Build history of the part. All positions in model axes, mm. Face numbers are marked on the shaded views. Give positions to 0.01 mm unless a question says otherwise; leave off trailing zeros. Order: outer loops, then holes, each group sorted by start corner. A loop starts at its lowest first (then second) coordinate and runs counter-clockwise, first axis right, second up. Notation, with made-up numbers: (36, 63) - (68, 63) arc R17 cw to (68, 89) - close; hole circle Ø6 at (-26, -2.5). An arc over 180 degrees is marked (long way). Answer in a Markdown table with one row per item.
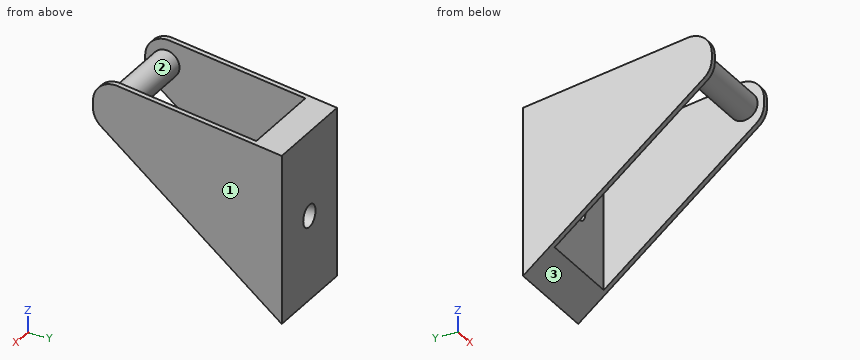
Autodesk Inventor part; units mm, degrees
ref_plane "YZ Plane" through (0, 0, 0) normal (1, 0, 0) x (0, 1, 0)
ref_plane "XZ Plane" through (0, 0, 0) normal (0, 1, 0) x (-1, 0, 0)
ref_plane "XY Plane" through (0, 0, 0) normal (0, 0, 1) x (1, 0, 0)
sketch "스케치1" plane through (0, 0, 0) normal (1, 0, 0) x (0, 1, 0)
  line L0 (-33.75, 41) -> (33.75, 41)
  line L1 (33.75, 41) -> (33.75, -41)
  line L2 (33.75, -41) -> (-33.75, -41)
  line L3 (-33.75, 29.5228) -> (-33.75, 32.1788)
  line L4 (-33.75, 41) -> (33.75, -41) construction
  line L5 (33.75, 41) -> (-33.75, -41) construction
  line L6 (33.75, 41) -> (33.75, 35)
  line L7 (33.75, 0) -> (33.75, 30)
  line L8 (33.75, 30) -> (-25.0437, 39.5812)
  line L9 (33.75, 0) -> (33.75, -30)
  line L10 (-31.0388, 23.7507) -> (33.75, -30)
  arc A0 (-33.75, 29.5228) -> (-31.0388, 23.7507) centre (-26.25, 29.5228) ccw
  arc A1 (-25.0437, 39.5812) -> (-33.75, 32.1788) centre (-26.25, 32.1788) ccw
  point P0 (0, 0)
  point P1 (-33.75, 26)
  dimension "d3" = 67.5
  dimension "d4" = 82
  dimension "d6" = 30
  dimension "d7" = 30
  dimension "d9" = 15
  dimension "d10" = 7.5
extrude "돌출1" add sketch "스케치1" along normal blind 36
ref_plane "작업 평면1" through (18, 0, 0) normal (1, 0, 0) x (0, 0, -1)
sketch "스케치2" plane through (18, 0, 0) normal (1, 0, 0) x (0, 0, -1)
  line L0 (-30, 33.75) -> (-39.5812, -25.0437)
  arc A0 (-39.5812, -25.0437) -> (-32.1788, -33.75) centre (-32.1788, -26.25) ccw
  line L1 (-32.1788, -33.75) -> (-29.5228, -33.75)
  arc A1 (-29.5228, -33.75) -> (-23.7507, -31.0388) centre (-29.5228, -26.25) ccw
  line L2 (-23.7507, -31.0388) -> (30, 33.75)
  line L3 (30, 33.75) -> (-30, 33.75)
  line L4 (30, 33.75) -> (-30, 33.75)
  line L5 (-30, 33.75) -> (-39.5812, -25.0437)
  circle A2 centre (-30.8508, -26.4664) radius 5
  line L6 (-30.8508, -26.4664) -> (-30.8508, 23.5336)
  line L7 (-30.8508, 23.5336) -> (21.5242, 23.5336)
  line L8 (-23.7507, -31.0388) -> (30, 33.75)
  line L9 (-30.8508, 23.5336) -> (-31.6649, 23.5336)
  point P0 (0, 0)
  dimension "d14" = 10
  dimension "d15" = 50
extrude "돌출2" cut sketch "스케치2" along normal blind 16 and the other way blind 16 contours L9 L7 L2 A1 L1 A0 L0
sketch "스케치3" plane through (0, 33.75, 30) normal (0, 1, 0) x (1, 0, 0)
  line L0 (0, 60) -> (0, 0)
  line L1 (0, 0) -> (36, 0)
  line L2 (36, 60) -> (36, 0)
  line L3 (0, 60) -> (36, 60)
  line L4 (18, 0) -> (18, 60)
  line L5 (0, 30) -> (36, 30)
  line L6 (36, 6.2493) -> (36, 60)
  circle A0 centre (18, 30) radius 4
  dimension "d20" = 8
extrude "돌출3" cut sketch "스케치3" against normal blind 16 contours A0 L4 L5 | L5 L4 A0 | A0 L5 L4 | L5 A0 L4
properties part number "Part_MetalLeg" material "스테인레스 스틸"
1. Cut at C-C on x = 18. Write the cut outline in (y, z).
Check result:
| item | result |
|---|---|
| outline | circle Ø10 at (-26.47, 30.85); (23.53, -21.52) - (33.75, -30) - (33.75, -4) - (23.53, -4) - close; (23.53, 4) - (33.75, 4) - (33.75, 30) - (23.53, 31.66) - close |
2. Probe line 1 (X direction, y = 10.5, z = 10); line 2 (X direction, y = 28, z = 0); line 3 (Y direction, x = 4.5, z = 2.5). List the from-to ranges inside material, lowest first.
Check result:
| item | result |
|---|---|
| line 1 | x = 0 to 2, 34 to 36 |
| line 2 | x = 0 to 14, 22 to 36 |
| line 3 | y = 23.53 to 33.75 |
3. Cut at D-D on y = -28. Write the cut outline in (x, z), and give its area (3 significant figures).
Check result:
| item | result |
|---|---|
| outline | (0, 21.23) - (2, 21.23) - (2, 26.09) - (34, 26.09) - (34, 21.23) - (36, 21.23) - (36, 39.47) - (34, 39.47) - (34, 35.61) - (2, 35.61) - (2, 39.47) - (0, 39.47) - close |
| area | 378 mm² |
4. Drop flat-ended pins along their axis: P1, Ø10.5, axis at x = 18, z = 0, coming from the +Y side; P2, Ø3, axis at x = 32, y = -22, coming from the +Z side. Give the stop position or say it passes through.
Check result:
| item | result |
|---|---|
| P1 | stops at y = 33.75 |
| P2 | stops at z = 34.88 |
5. Two-plate mould, pull along X, no slides. Class the marked faces 1, 2 and 3: +X half, -X half, draft (parallel to the pull), parting line (faces both ways), or undercut.
Check result:
| item | result |
|---|---|
| face 1 | +X half |
| face 2 | undercut |
| face 3 | draft |
6. Cut at A-A on y = 9.5. Write the cut outline in (x, z), and give its area (3 significant figures).
Check result:
| item | result |
|---|---|
| outline | (0, -9.88) - (2, -9.88) - (2, 33.95) - (0, 33.95) - close; (34, -9.88) - (36, -9.88) - (36, 33.95) - (34, 33.95) - close |
| area | 175 mm² |
7. Cut at B-B on z = -2. Write the cut outline in (x, y), and give its area (3 significant figures).
Check result:
| item | result |
|---|---|
| outline | (0, 0) - (2, 0) - (2, 23.53) - (14.54, 23.53) - (14.54, 33.75) - (0, 33.75) - close; (21.46, 23.53) - (34, 23.53) - (34, 0) - (36, 0) - (36, 33.75) - (21.46, 33.75) - close |
| area | 391 mm² |
